from build123d import *

# Parameters (mm, degrees)
SKETCH_1_R          = 10.65
SKETCH_1_R_2        = 8.65
EXTRUDE_1_DEPTH     = 150
SKETCH_2_R          = 3.1
CUT_EXTRUDE_1_DEPTH = 5
OTHER_START         = -3
OTHER_1_DEPTH       = 3


# Read off the part's stored shape, not the designer's step: Полость1
with BuildPart() as part:
    # Эскиз1 → Бобышка-Вытянуть1 (new body)
    with BuildSketch(Plane(origin=(0, 0, 0), x_dir=(1, 0, 0), z_dir=(0, 1, 0))):
        with Locations(Location((0, 0, 0), (0, 0, 270))):
            Circle(SKETCH_1_R)
        with Locations(Location((0, 0, 0), (0, 0, 270))):
            Circle(SKETCH_1_R_2, mode=Mode.SUBTRACT)
    extrude(amount=-EXTRUDE_1_DEPTH)

    # Эскиз2 → Вырез-Вытянуть1 (cut, symmetric)
    with BuildSketch(Plane(origin=(8.65, 0, 0), x_dir=(0, 0, -1), z_dir=(1, 0, 0))):
        with Locations((0, -7)):
            Circle(SKETCH_2_R)
    extrude(amount=CUT_EXTRUDE_1_DEPTH, both=True, mode=Mode.SUBTRACT)

    # Полость1 outline → Полость1 (cut)
    with BuildSketch(Plane(origin=(0, 0, 0), x_dir=(1, 0, 0), z_dir=(0, 1, 0)).offset(OTHER_START)):
        with BuildLine():
            Line((10.141991915, -3.25), (8.01623353, -3.25))
            ThreePointArc((8.01623353, -3.25), (6.673866727, -5.502908587), (4.718050445, -7.25))
            Line((4.718050445, -7.25), (7.801281946, -7.25))
            ThreePointArc((7.801281946, -7.25), (9.191858855, -5.378868914), (10.141991915, -3.25))
        make_face()
        with BuildLine():
            Line((-7.801281946, -7.25), (-4.718050445, -7.25))
            ThreePointArc((-4.718050445, -7.25), (-6.673866727, -5.502908587), (-8.01623353, -3.25))
            Line((-8.01623353, -3.25), (-10.141991915, -3.25))
            ThreePointArc((-10.141991915, -3.25), (-9.191858855, -5.378868914), (-7.801281946, -7.25))
        make_face()
    other_1 = extrude(amount=OTHER_1_DEPTH, mode=Mode.SUBTRACT)

    # Зеркальное отражение1: Полость1 across plane
    add(other_1.mirror(Plane.XY), mode=Mode.SUBTRACT)


solid = part.part
Design review of the part built by this model. Coordinates are the model's own, in mm. A direction names the side the tool comes from. Coordinates: 2 decimals unless noted, no trailing zeros. Order: outer loops, then holes, each group sorted by start corner. A loop starts at its lowest first (then second) coordinate and runs counter-clockwise, first axis right, second up. Notation, with made-up numbers: (-31.75, -36.75) -> (10.25, -36.75) arc R12 cw to (10.25, -19.75) -> close; hole circle Ø11 at (7, -31.75). An arc over 180 degrees is marked (long way). One line per item, written item: value.
1) We need section C-C, the plane z = -6. Give the boundary of the cut face in (x, y).
Output values:
outline: (-8.8, -150) -> (-6.23, -150) -> (-6.23, -3) -> (-8.8, -3) -> close; (6.23, -150) -> (8.8, -150) -> (8.8, -3) -> (6.23, -3) -> close
2) We need section B-B, the plane x = 6.25. Give the boundary of the cut face in (y, z).
Output values:
outline: (-150, -8.62) -> (0, -8.62) -> (0, -7.25) -> (-3, -7.25) -> (-3, -5.98) -> (-150, -5.98) -> close; (-150, 5.98) -> (-3, 5.98) -> (-3, 7.25) -> (0, 7.25) -> (0, 8.62) -> (-150, 8.62) -> close
3) Draft analysis for pull direction Z (two halves, no side actions). For faces 3 (the face through (9, 0, 0)), 4 (the face through (-6, -2, 7.25)), 5 (the face through (-10.4, -74, -2.3)), 6 (the face through (9.384, -8.187, -2.864)), state which applies: +Z half, -Z half, draft (parallel to the pull), parting line (faces both ways), or undercut.
Output values:
face 3: draft
face 4: undercut
face 5: parting line
face 6: undercut
4) We need section D-D, the plane y = -128. Give the boundary of the cut face in (x, z).
Output values:
outline: circle Ø21.3 at (0, 0); hole circle Ø17.3 at (0, 0)
5) We need section A-A, the plane z = 0. Give the boundary of the cut face in (x, y), then the cut area to 3 significant figures.
Output values:
outline: (-10.65, -150) -> (-8.65, -150) -> (-8.65, 0) -> (-10.65, 0) -> close; (8.65, -150) -> (10.65, -150) -> (10.65, -10.1) -> (8.65, -10.1) -> close; (8.65, -3.9) -> (10.65, -3.9) -> (10.65, 0) -> (8.65, 0) -> close
area: 588 mm2
6) Machinability: for faces 1 (the face through (-7.674, -73.95, 3.991)), 2 (the face through (6, -2, 7.25)), which of the approach directions +Z, -Z, +X, -X, +Y, -Y give a long, thin tool a straight path to every point of the face, cutting with its end or side? Answer none if there is none.
Output values:
face 1: +Y, -Y
face 2: +X, -X, +Y
7) Clearance check with flat-ended pins moving along their axes: P1, Ø10.5, axis at x = 0, z = 0, coming from the -Y side; P2, Ø2.5, axis at x = 9, y = -2, coming from the +Z side; P3, Ø2.5, axis at x = -9, y = -1.5, coming from the -Z side; P4, Ø0.6, axis at x = -9.5, y = -2, coming from the +Z side. State where each tip first meets the part, or that it passes through.
Output values:
P1: passes through
P2: stops at z = 7.3
P3: stops at z = -7.3
P4: stops at z = 3.25
8) To check wall thickness, follow probe 1 along X at (y, z) = (-90, 0); probe 2 along Y at (x, z) = (9.4, 0); probe 3 along Z at (x, y) = (0.5, -98). State the ranges of each line that lie inside material, in increasing order. Write a range as [from, to].
Output values:
probe 1: x = [-10.65, -8.65], [8.65, 10.65]
probe 2: y = [-150, -10.1], [-3.9, 0]
probe 3: z = [-10.64, -8.64], [8.64, 10.64]
